The model under review builds one solid part; all positions refer to its coordinate system, in mm. Face numbers are marked on the shaded views. A direction names the side the tool comes from. Coordinates: 2 decimals unless noted, no trailing zeros. Order: outer loops, then holes, each group sorted by start corner. A loop starts at its lowest first (then second) coordinate and runs counter-clockwise, first axis right, second up. Notation, with made-up numbers: M -24.75,-20 L 24.25,-20 A19 ccw 24.25,3 Z; hole C 61.25,-32 d7. An arc over 180 degrees is marked long. Answer as CSV lines item,"result". Start each with the question number.
Q1. Consider section D-D on z = -1. Write out the cut boundary in (x, y), and give its area (3 significant figures).
Q2. For P1, Ø1.5, axis at y = -3.5, z = -1.5, coming from the +X side; P2, Ø3.5, axis at x = -12.5, z = -10.5, coming from the +Y side; P3, Ø3, axis at x = 8, z = -15.5, coming from the +Y side; P4, Ø0.7, axis at x = 10, y = -1.5, coming from the -Z side, all flat-tipped, find the tip position at first contact; note any pin that passes through.
Q3. The part is to be moulded in two halves that separate along X. For the marked faces 1, 2 and 3, say which applies: +X half, -X half, draft (parallel to the pull), parting line (faces both ways), or undercut.
Q4. Consider section C-C on x = -0.5. Write out the cut boundary in (y, z), and give its area (3 significant figures).
Q5. Consider section A-A on y = -1.8. Write out the cut boundary in (x, z).
Q6. Machinability: for the marked faces 4, 5 and 6, which of the approach directions +Z, -Z, +X, -X, +Y, -Y give a long, thin tool a straight path to every point of the face, cutting with its end or side? Answer none if there is none.
Q7. Wall thickness on L1, parallel to X at y = -3.55, z = -8; L2, parallel to X at y = -0.2, z = -9.25; L3, parallel to Y at x = 5.25, z = -9.75: over which ranges is each line inside the solid? List them lowest first. Write a range as [from, to].
Q8. Consider section B-B on z = -15.5. Write out the cut boundary in (x, y).
from build123d import *

# Parameters (mm, degrees)
BASE_FLANGE1_DEPTH              = 0.3
EDGE_FLANGE2_DEPTH              = 7.6
EDGE_FLANGE3_DEPTH              = 7.4
EDGE_FLANGE3_BEND_DEPTH         = 7.4
EDGE_FLANGE9_STRIP_W            = 1.8
EDGE_FLANGE9_STRIP_H            = 0.3
EDGE_FLANGE9_STRIP_CUT_DEPTH    = 5.1
EDGE_FLANGE9_RELIEF_W           = 1.95
EDGE_FLANGE9_RELIEF_H           = 0.15
EDGE_FLANGE9_RELIEF_CUT_DEPTH   = 0.3
EDGE_FLANGE9_STRIP_2_W          = 1.8
EDGE_FLANGE9_STRIP_2_H          = 0.3
EDGE_FLANGE9_STRIP_CUT_2_DEPTH  = 5.1
EDGE_FLANGE9_RELIEF_2_W         = 1.95
EDGE_FLANGE9_RELIEF_2_H         = 0.15
EDGE_FLANGE9_RELIEF_CUT_2_DEPTH = 0.3
EDGE_FLANGE9_DEPTH              = 5.1
EDGE_FLANGE9_BEND_DEPTH         = 5.1
SKETCH164_R                     = 3.1
CUT_EXTRUDE1_DEPTH              = 10
CUT_EXTRUDE2_DEPTH              = 26.150701614
CUT_EXTRUDE2_DEPTH_BACK         = 26.150701614
SKETCH228_W                     = 2.9
SKETCH228_H                     = 7.24828594
EDGE_FLANGE10_DEPTH             = 2.5
EDGE_FLANGE10_BEND_DEPTH        = 2.5
EDGE_FLANGE11_STRIP_CUT_DEPTH   = 2.5
EDGE_FLANGE11_STRIP_CUT_2_DEPTH = 2.5
EDGE_FLANGE11_DEPTH             = 2.5
EDGE_FLANGE11_BEND_DEPTH        = 2.5
BREAK_CORNER1_START             = -1.168240888
BREAK_CORNER1_DEPTH             = 0.3


# Read off the part's stored shape, not the designer's step: Break-Corner1
# Sheet-metal steps are written as plain solids
with BuildPart() as part:
    # Sketch1 → Base-Flange1 (new body)
    with BuildSketch(Plane(origin=(0, 0, 0), x_dir=(1, 0, 0), z_dir=(0, 1, 0))):
        with BuildLine():
            Line((-3.8, 0), (3.8, 0))
            Line((3.8, 0), (9.95, 6.15))
            Line((9.95, 6.15), (9.95, 16.8))
            ThreePointArc((9.95, 16.8), (8.121537451, 19.561792896), (4.865, 18.957029207))
            ThreePointArc((4.865, 18.957029207), (0, 16.990097357), (-4.865, 18.957029207))
            ThreePointArc((-4.865, 18.957029207), (-8.121537451, 19.561792896), (-9.95, 16.8))
            Line((-9.95, 16.8), (-9.95, 6.15))
            Line((-9.95, 6.15), (-3.8, 0))
        make_face()
    extrude(amount=-BASE_FLANGE1_DEPTH)

    # Edge-Flange2 section (across the edge) → Edge-Flange2 (add)
    with BuildSketch(Plane(origin=(3.8, -0.3, 0.3), x_dir=(0, 0, -1), z_dir=(-1, 0, 0))):
        with BuildLine():
            Line((-0.3, 0.3), (-0.3, 3))
            Line((-0.3, 3), (0, 3))
            Line((0, 3), (0, 0.3))
            ThreePointArc((0, 0.3), (0.087867966, 0.087867966), (0.3, 0))
            Line((0.3, 0), (0.3, -0.3))
            ThreePointArc((0.3, -0.3), (-0.124264069, -0.124264069), (-0.3, 0.3))
        make_face()
    extrude(amount=EDGE_FLANGE2_DEPTH)

    # Edge-Flange3 section (across the edge) → Edge-Flange3 (add)
    with BuildSketch(Plane(origin=(10.25, -0.3, -13.55), x_dir=(-1, 0, 0), z_dir=(0, 0, 1))):
        with BuildLine():
            Line((-0.3, 0.3), (-0.3, 3.8249596))
            Line((-0.3, 3.8249596), (0, 3.8249596))
            Line((0, 3.8249596), (0, 0.3))
            ThreePointArc((0, 0.3), (0.087867966, 0.087867966), (0.3, 0))
            Line((0.3, 0), (0.3, -0.3))
            ThreePointArc((0.3, -0.3), (-0.124264069, -0.124264069), (-0.3, 0.3))
        make_face()
    extrude(amount=EDGE_FLANGE3_DEPTH)

    # Edge-Flange3 section 2 (across the edge) → Edge-Flange3 bend (add)
    with BuildSketch(Plane(origin=(-10.25, -0.3, -6.15), x_dir=(1, 0, 0), z_dir=(0, 0, -1))):
        with BuildLine():
            Line((-0.3, 0.3), (-0.3, 3.8249596))
            Line((-0.3, 3.8249596), (0, 3.8249596))
            Line((0, 3.8249596), (0, 0.3))
            ThreePointArc((0, 0.3), (0.087867966, 0.087867966), (0.3, 0))
            Line((0.3, 0), (0.3, -0.3))
            ThreePointArc((0.3, -0.3), (-0.124264069, -0.124264069), (-0.3, 0.3))
        make_face()
    extrude(amount=EDGE_FLANGE3_BEND_DEPTH)

    # Edge-Flange9 strip (across the edge) → Edge-Flange9 strip cut (cut)
    with BuildSketch(Plane(origin=(-10.55, -4.1249596, -12.4), x_dir=(0, 1, 0), z_dir=(0, 0, 1))):
        with Locations((-0.3, -0.15)):
            Rectangle(EDGE_FLANGE9_STRIP_W, EDGE_FLANGE9_STRIP_H)
    extrude(amount=EDGE_FLANGE9_STRIP_CUT_DEPTH, mode=Mode.SUBTRACT)

    # Edge-Flange9 relief (on the sheet) → Edge-Flange9 relief cut (cut)
    with BuildSketch(Plane(origin=(-10.55, -3.5249596, -12.4), x_dir=(0, 1, 0), z_dir=(-1, 0, 0))):
        with Locations((-0.825, 0.075)):
            Rectangle(EDGE_FLANGE9_RELIEF_W, EDGE_FLANGE9_RELIEF_H)
        with Locations((-0.825, -5.175)):
            Rectangle(EDGE_FLANGE9_RELIEF_W, EDGE_FLANGE9_RELIEF_H)
    extrude(amount=-EDGE_FLANGE9_RELIEF_CUT_DEPTH, mode=Mode.SUBTRACT)

    # Edge-Flange9 strip 2 (across the edge) → Edge-Flange9 strip cut 2 (cut)
    with BuildSketch(Plane(origin=(10.55, -4.1249596, -7.3), x_dir=(0, 1, 0), z_dir=(0, 0, -1))):
        with Locations((-0.3, -0.15)):
            Rectangle(EDGE_FLANGE9_STRIP_2_W, EDGE_FLANGE9_STRIP_2_H)
    extrude(amount=EDGE_FLANGE9_STRIP_CUT_2_DEPTH, mode=Mode.SUBTRACT)

    # Edge-Flange9 relief 2 (on the sheet) → Edge-Flange9 relief cut 2 (cut)
    with BuildSketch(Plane(origin=(10.55, -3.5249596, -7.3), x_dir=(0, 1, 0), z_dir=(1, 0, 0))):
        with Locations((-0.825, 0.075)):
            Rectangle(EDGE_FLANGE9_RELIEF_2_W, EDGE_FLANGE9_RELIEF_2_H)
        with Locations((-0.825, -5.175)):
            Rectangle(EDGE_FLANGE9_RELIEF_2_W, EDGE_FLANGE9_RELIEF_2_H)
    extrude(amount=-EDGE_FLANGE9_RELIEF_CUT_2_DEPTH, mode=Mode.SUBTRACT)

    # Edge-Flange9 section (across the edge) → Edge-Flange9 (add)
    with BuildSketch(Plane(origin=(-10.55, -4.1249596, -12.4), x_dir=(0, 1, 0), z_dir=(0, 0, 1))):
        with BuildLine():
            Line((0, 0.3), (0, 4.4))
            Line((0, 4.4), (0.3, 4.4))
            Line((0.3, 4.4), (0.3, 0.3))
            ThreePointArc((0.3, 0.3), (0.387867966, 0.087867966), (0.6, 0))
            Line((0.6, 0), (0.6, -0.3))
            ThreePointArc((0.6, -0.3), (0.175735931, -0.124264069), (0, 0.3))
        make_face()
    extrude(amount=EDGE_FLANGE9_DEPTH)

    # Edge-Flange9 section 2 (across the edge) → Edge-Flange9 bend (add)
    with BuildSketch(Plane(origin=(10.55, -4.1249596, -7.3), x_dir=(0, 1, 0), z_dir=(0, 0, -1))):
        with BuildLine():
            Line((0, 0.3), (0, 4.4))
            Line((0, 4.4), (0.3, 4.4))
            Line((0.3, 4.4), (0.3, 0.3))
            ThreePointArc((0.3, 0.3), (0.387867966, 0.087867966), (0.6, 0))
            Line((0.6, 0), (0.6, -0.3))
            ThreePointArc((0.6, -0.3), (0.175735931, -0.124264069), (0, 0.3))
        make_face()
    extrude(amount=EDGE_FLANGE9_BEND_DEPTH)

    # Sketch164 → Cut-Extrude1 (cut)
    with BuildSketch(Plane(origin=(0, 0, 0), x_dir=(1, 0, 0), z_dir=(0, 1, 0))):
        with Locations(Location((-5.5, 9.25, 0), (0, 0, 270))):
            Circle(SKETCH164_R)
        with Locations(Location((5.5, 9.25, 0), (0, 0, 270))):
            Circle(SKETCH164_R)
    extrude(amount=-CUT_EXTRUDE1_DEPTH, mode=Mode.SUBTRACT)

    # Sketch228 → Cut-Extrude2 (cut, two sides: drawn at the far end of the back side and taken through both)
    with BuildSketch(Plane(origin=(0, 0, 0), x_dir=(1, 0, 0), z_dir=(0, 1, 0)).offset(-CUT_EXTRUDE2_DEPTH_BACK)):
        with Locations((-5.5, 13.17585703)):
            Rectangle(SKETCH228_W, SKETCH228_H)
        with Locations((5.5, 13.17585703)):
            Rectangle(SKETCH228_W, SKETCH228_H)
    extrude(amount=CUT_EXTRUDE2_DEPTH + CUT_EXTRUDE2_DEPTH_BACK, mode=Mode.SUBTRACT)

    # Edge-Flange10 section (across the edge) → Edge-Flange10 (add)
    with BuildSketch(Plane(origin=(-4.25, -0.3, -16.773753401), x_dir=(0, -0.9848077530122092, -0.1736481776669237), z_dir=(-1, 0, 0))):
        with BuildLine():
            Line((-0.3, 0.026246599), (-0.3, 4.973753401))
            Line((-0.3, 4.973753401), (0, 4.973753401))
            Line((0, 4.973753401), (0, 0.026246599))
            ThreePointArc((0, 0.026246599), (0.001141591, 9.9876e-05), (0.004557674, -0.025847854))
            Line((0.004557674, -0.025847854), (-0.290884652, -0.077942308))
            ThreePointArc((-0.290884652, -0.077942308), (-0.297716819, -0.026046847), (-0.3, 0.026246599))
        make_face()
    extrude(amount=EDGE_FLANGE10_DEPTH)

    # Edge-Flange10 section 2 (across the edge) → Edge-Flange10 bend (add)
    with BuildSketch(Plane(origin=(6.75, -0.3, -16.773753401), x_dir=(0, -0.9848077530122092, -0.1736481776669237), z_dir=(-1, 0, 0))):
        with BuildLine():
            Line((-0.3, 0.026246599), (-0.3, 4.973753401))
            Line((-0.3, 4.973753401), (0, 4.973753401))
            Line((0, 4.973753401), (0, 0.026246599))
            ThreePointArc((0, 0.026246599), (0.001141591, 9.9876e-05), (0.004557674, -0.025847854))
            Line((0.004557674, -0.025847854), (-0.290884652, -0.077942308))
            ThreePointArc((-0.290884652, -0.077942308), (-0.297716819, -0.026046847), (-0.3, 0.026246599))
        make_face()
    extrude(amount=EDGE_FLANGE10_BEND_DEPTH)

    # Edge-Flange11 strip (across the edge) → Edge-Flange11 strip cut (cut)
    with BuildSketch(Plane(origin=(-6.75, -0.868240888, -11.823468037), x_dir=(0, 1, 0), z_dir=(1, 0, 0))):
        Polygon((-0.603451372, 1.694711648), (-0.290884652, -0.077942308), (0.004557674, -0.025847854), (-0.308009046, 1.746806101), align=None)
    extrude(amount=EDGE_FLANGE11_STRIP_CUT_DEPTH, mode=Mode.SUBTRACT)

    # Edge-Flange11 strip 2 (across the edge) → Edge-Flange11 strip cut 2 (cut)
    with BuildSketch(Plane(origin=(4.25, -0.868240888, -11.823468037), x_dir=(0, 1, 0), z_dir=(1, 0, 0))):
        Polygon((-0.603451372, 1.694711648), (-0.290884652, -0.077942308), (0.004557674, -0.025847854), (-0.308009046, 1.746806101), align=None)
    extrude(amount=EDGE_FLANGE11_STRIP_CUT_2_DEPTH, mode=Mode.SUBTRACT)

    # Edge-Flange11 section (across the edge) → Edge-Flange11 (add)
    with BuildSketch(Plane(origin=(-6.75, -0.868240888, -11.823468037), x_dir=(0, 1, 0), z_dir=(1, 0, 0))):
        with BuildLine():
            Line((-0.3, 0.026246599), (-0.3, 2.973753401))
            Line((-0.3, 2.973753401), (0, 2.973753401))
            Line((0, 2.973753401), (0, 0.026246599))
            ThreePointArc((0, 0.026246599), (0.001141591, 9.9876e-05), (0.004557674, -0.025847854))
            Line((0.004557674, -0.025847854), (-0.290884652, -0.077942308))
            ThreePointArc((-0.290884652, -0.077942308), (-0.297716819, -0.026046847), (-0.3, 0.026246599))
        make_face()
    extrude(amount=EDGE_FLANGE11_DEPTH)

    # Edge-Flange11 section 2 (across the edge) → Edge-Flange11 bend (add)
    with BuildSketch(Plane(origin=(4.25, -0.868240888, -11.823468037), x_dir=(0, 1, 0), z_dir=(1, 0, 0))):
        with BuildLine():
            Line((-0.3, 0.026246599), (-0.3, 2.973753401))
            Line((-0.3, 2.973753401), (0, 2.973753401))
            Line((0, 2.973753401), (0, 0.026246599))
            ThreePointArc((0, 0.026246599), (0.001141591, 9.9876e-05), (0.004557674, -0.025847854))
            Line((0.004557674, -0.025847854), (-0.290884652, -0.077942308))
            ThreePointArc((-0.290884652, -0.077942308), (-0.297716819, -0.026046847), (-0.3, 0.026246599))
        make_face()
    extrude(amount=EDGE_FLANGE11_BEND_DEPTH)

    # Break-Corner1 outline → Break-Corner1 (cut)
    with BuildSketch(Plane(origin=(0, 0, 0), x_dir=(1, 0, 0), z_dir=(0, 1, 0)).offset(BREAK_CORNER1_START)):
        with BuildLine():
            ThreePointArc((6.75, 9.849714636), (6.457106781, 9.142607855), (5.75, 8.849714636))
            Line((5.75, 8.849714636), (6.75, 8.849714636))
            Line((6.75, 8.849714636), (6.75, 9.849714636))
        make_face()
        with BuildLine():
            Line((4.25, 8.849714636), (5.25, 8.849714636))
            ThreePointArc((5.25, 8.849714636), (4.542893219, 9.142607855), (4.25, 9.849714636))
            Line((4.25, 9.849714636), (4.25, 8.849714636))
        make_face()
        with BuildLine():
            ThreePointArc((-4.25, 9.849714636), (-4.542893219, 9.142607855), (-5.25, 8.849714636))
            Line((-5.25, 8.849714636), (-4.25, 8.849714636))
            Line((-4.25, 8.849714636), (-4.25, 9.849714636))
        make_face()
        with BuildLine():
            ThreePointArc((-5.75, 8.849714636), (-6.457106781, 9.142607855), (-6.75, 9.849714636))
            Line((-6.75, 9.849714636), (-6.75, 8.849714636))
            Line((-6.75, 8.849714636), (-5.75, 8.849714636))
        make_face()
    extrude(amount=BREAK_CORNER1_DEPTH, mode=Mode.SUBTRACT)


solid = part.part
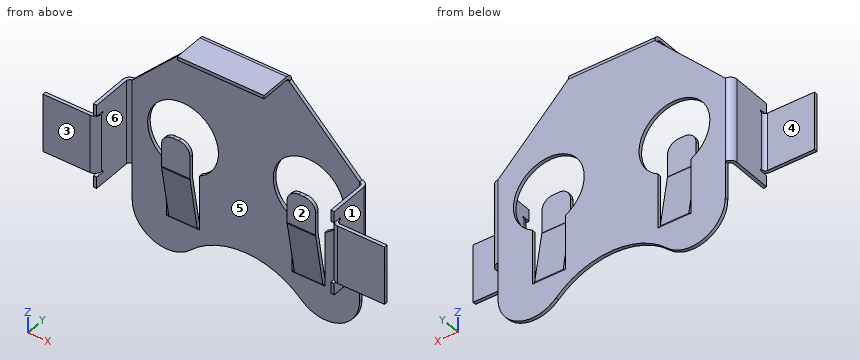
Evaluation:
1,outline,"M -4.8,-0.3 L 4.8,-0.3 L 4.8,0 L -4.8,0 Z"
1,area,"2.88 mm²"
2,P1,"passes through"
2,P2,"stops at y = -3.81"
2,P3,"stops at y = 0"
2,P4,"stops at z = -13.55"
3,face 1,"+X half"
3,face 2,"undercut"
3,face 3,"draft"
4,outline,"M -3.3,0.3 L -0.6,0.3 A0.3 cw -0.3,0 L -0.3,-17.01 L 0,-17.01 L 0,0 A0.6 ccw -0.6,0.6 L -3.3,0.6 Z"
4,area,"6.12 mm²"
5,outline,"M -10.55,-13.55 L -10.25,-13.55 L -10.25,-6.15 L -10.55,-6.15 Z; M -3.8,0.3 L 3.8,0.3 L 3.8,0.6 L -3.8,0.6 Z; M 10.25,-13.55 L 10.55,-13.55 L 10.55,-6.15 L 10.25,-6.15 Z"
6,face 4,"+Z, -Z, -X, +Y"
6,face 5,"-Y"
6,face 6,"+Z, -Z, -Y"
7,L1,"x = [-10.55, -10.25], [10.25, 10.55]"
7,L2,"x = [-10.4, -8.6], [-2.4, 2.4], [8.6, 10.4]"
7,L3,"y = [-1.17, -0.87]"
8,outline,"M -9.95,-0.3 L -6.95,-0.3 L -6.95,0 L -9.95,0 Z; M -6.75,-0.52 L -4.25,-0.52 L -4.25,-0.22 L -6.75,-0.22 Z; M -4.05,-0.3 L 4.05,-0.3 L 4.05,0 L -4.05,0 Z; M 4.25,-0.52 L 6.75,-0.52 L 6.75,-0.22 L 4.25,-0.22 Z; M 6.95,-0.3 L 9.95,-0.3 L 9.95,0 L 6.95,0 Z"
